Work out the finished part from the listing and answer in its coordinate system (mm). A direction names the side the tool comes from. Coordinates: 2 decimals unless noted, no trailing zeros. Order: outer loops, then holes, each group sorted by start corner. A loop starts at its lowest first (then second) coordinate and runs counter-clockwise, first axis right, second up. Notation, with made-up numbers: M 17.5,15 L 63.5,15 A19 ccw 63.5,23 Z; hole C -23.75,50.5 d11. An arc over 180 degrees is marked long. Write item = value, one per line. Start each with the question number.
Q1. Find section D-D on z = 42. Give the vertices of the cut face in (x, y), and give its area (3 significant figures).
Q2. Determine the mould class of faces 4 (the flat face through (21, 67, 30)), 5 (the flat face through (112, 35, 40)), 6 (the cylindrical face through (49.993, 60.66, 44.79)) for opening direction X: released by +X, released by -X, zero draft, split by the parting line, or undercut.
Q3. Straight lines are drawn through the part: line 1 along Y through (x, z) = (110, 7.25); line 2 along Y through (x, z) = (80, 66.75); line 3 along Y through (x, z) = (110, 24.5). For each, find the intervals that lie inside material, in ascending order.
Q4. Find section B-B on x = 30. Give the vertices of the cut face in (y, z), and give its area (3 significant figures).
Q5. Each of these flat-tipped pins is pushed along its axis until it touches: P1, Ø22, axis at x = 114.5, y = 28.5, coming from the -Z side; P2, Ø10, axis at x = 116, z = 15.5, coming from the +Y side; P3, Ø3, axis at x = 87, z = 70.5, coming from the -Y side; P4, Ø18, axis at x = 30, y = 60, coming from the +Z side. Where does it stop, or does it pass through?
Q6. Find section C-C on y = 93. Give the vertices of the cut face in (x, z), and give its area (3 significant figures).
Q7. A tool of negligible diameter and unlimited length cuts with its end or side. For faces 1 (the cylindrical face through (102, 24, 50)), 2 (the flat face through (8, 30, 37)), 3 (the flat face through (112, 95, 20)), from which of +Z, -Z, +X, -X, +Y, -Y can it reach the whole face along a straight path? Write none if from no direction.
Q8. Find section A-A on z = 57.5. Give the vertices of the cut face in (x, y), and give its area (3 significant figures).
```python
from build123d import *

# Parameters (mm, degrees)
SKETCH1_W                  = 140
SKETCH1_H                  = 120
BOSS_EXTRUDE1_DEPTH        = 60
SKETCH2_W                  = 10
SKETCH2_H                  = 60
CUT_EXTRUDE1_DEPTH         = 60
CUT_EXTRUDE2_DEPTH         = 60
SKETCH4_R                  = 10
CUT_EXTRUDE3_DEPTH         = 60
SKETCH5_R                  = 10
CUT_EXTRUDE4_DEPTH         = 60
SKETCH6_R                  = 10
CUT_EXTRUDE5_DEPTH         = 60
SKETCH7_R                  = 5
CUT_EXTRUDE6_DEPTH         = 60
SKETCH8_R                  = 10
CUT_EXTRUDE7_DEPTH         = 20
SKETCH9_R                  = 5
CUT_EXTRUDE8_DEPTH         = 47
SKETCH10_R                 = 10
CUT_EXTRUDE9_DEPTH         = 20
SKETCH11_R                 = 20
BOSS_EXTRUDE2_DEPTH        = 20
F_20_0MM_DOWEL_HOLE1_D     = 20
F_20_0MM_DOWEL_HOLE1_DEPTH = 30
F_20_0MM_DOWEL_HOLE1_TIP   = 6.00860619


with BuildPart() as part:
    # Sketch1 → Boss-Extrude1 (new body)
    with BuildSketch(Plane.XY):
        with Locations((70, 60)):
            Rectangle(SKETCH1_W, SKETCH1_H)
    extrude(amount=BOSS_EXTRUDE1_DEPTH)

    # Sketch2 → Cut-Extrude1 (cut)
    with BuildSketch(Plane.XY.offset(60)):
        with BuildLine():
            Line((140, 120), (80, 120))
            ThreePointArc((80, 120), (122.426406871, 102.426406871), (140, 60))
            Line((140, 60), (140, 120))
        make_face()
        with BuildLine():
            Line((140, 0), (140, 60))
            ThreePointArc((140, 60), (122.426406871, 17.573593129), (80, 0))
            Line((80, 0), (140, 0))
        make_face()
        with Locations((5, 60)):
            Rectangle(SKETCH2_W, SKETCH2_H)
    extrude(amount=-CUT_EXTRUDE1_DEPTH, mode=Mode.SUBTRACT)

    # Sketch3 → Cut-Extrude2 (cut)
    with BuildSketch(Plane.XY.offset(30)):
        with BuildLine():
            ThreePointArc((20, 90), (50, 60), (20, 30))
            Line((20, 30), (10, 30))
            Line((10, 30), (10, 90))
            Line((10, 90), (20, 90))
        make_face()
    extrude(amount=CUT_EXTRUDE2_DEPTH, mode=Mode.SUBTRACT)

    # Sketch4 → Cut-Extrude3 (cut)
    with BuildSketch(Plane.XY.offset(30)):
        with Locations((30, 60)):
            Circle(SKETCH4_R)
    extrude(amount=-CUT_EXTRUDE3_DEPTH, mode=Mode.SUBTRACT)

    # Sketch5 → Cut-Extrude4 (cut)
    with BuildSketch(Plane.XY.offset(20)):
        with Locations((110, 90)):
            Circle(SKETCH5_R)
    extrude(amount=-CUT_EXTRUDE4_DEPTH, mode=Mode.SUBTRACT)

    # Sketch6 → Cut-Extrude5 (cut)
    with BuildSketch(Plane.XY.offset(40)):
        with Locations((110, 90)):
            Circle(SKETCH6_R)
    extrude(amount=CUT_EXTRUDE5_DEPTH, mode=Mode.SUBTRACT)

    # Sketch7 → Cut-Extrude6 (cut)
    with BuildSketch(Plane.XY.offset(40)):
        with Locations((110, 90)):
            Circle(SKETCH7_R)
    extrude(amount=-CUT_EXTRUDE6_DEPTH, mode=Mode.SUBTRACT)

    # Sketch8 → Cut-Extrude7 (cut)
    with BuildSketch(Plane.XY.offset(60)):
        with Locations((110, 30)):
            Circle(SKETCH8_R)
    extrude(amount=-CUT_EXTRUDE7_DEPTH, mode=Mode.SUBTRACT)

    # Sketch9 → Cut-Extrude8 (cut)
    with BuildSketch(Plane.XY.offset(40)):
        with Locations((110, 30)):
            Circle(SKETCH9_R)
    extrude(amount=-CUT_EXTRUDE8_DEPTH, mode=Mode.SUBTRACT)

    # Sketch10 → Cut-Extrude9 (cut)
    with BuildSketch(Plane(origin=(0, 0, 0), x_dir=(-1, 0, 0), z_dir=(0, 0, -1))):
        with Locations((-110, 30)):
            Circle(SKETCH10_R)
    extrude(amount=-CUT_EXTRUDE9_DEPTH, mode=Mode.SUBTRACT)

    # Sketch11 → Boss-Extrude2 (add)
    with BuildSketch(Plane.XY.offset(60)):
        with Locations((80, 60)):
            Circle(SKETCH11_R)
    extrude(amount=BOSS_EXTRUDE2_DEPTH)

    # Ø20.0mm Dowel Hole1
    with Locations(Plane(origin=(80, 60, 80), x_dir=(1, 0, 0), z_dir=(0, 0, 1))):
        with Locations((0, 0)):
            Hole(F_20_0MM_DOWEL_HOLE1_D / 2, depth=F_20_0MM_DOWEL_HOLE1_DEPTH)
            with Locations((0, 0, -(F_20_0MM_DOWEL_HOLE1_DEPTH + F_20_0MM_DOWEL_HOLE1_TIP / 2))):  # 118° drill point
                Cone(0, F_20_0MM_DOWEL_HOLE1_D / 2, F_20_0MM_DOWEL_HOLE1_TIP, mode=Mode.SUBTRACT)


solid = part.part
```
Findings below:
q1.outline = M 0,0 L 80,0 A60 ccw 80,120 L 0,120 L 0,90 L 20,90 A30 cw 20,30 L 0,30 Z; hole C 110,30 d20; hole C 110,90 d20
q1.area = 12,000 mm^2
q2.face_4 = zero draft
q2.face_5 = undercut
q2.face_6 = released by -X
q3.line_1 = 8.04 to 20, 40 to 80, 100 to 111.96
q3.line_2 = 40 to 50, 70 to 80
q3.line_3 = 8.04 to 25, 35 to 85, 95 to 111.96
q4.outline = M 0,0 L 50,0 L 50,30 L 31.72,30 L 31.72,60 L 0,60 Z; M 70,0 L 120,0 L 120,60 L 88.28,60 L 88.28,30 L 70,30 Z
q4.area = 4,900 mm^2
q5.P1 = 0
q5.P2 = 111.37
q5.P3 = 40.77
q5.P4 = through
q6.outline = M 0,0 L 100.46,0 L 100.46,20 L 106,20 L 106,40 L 100.46,40 L 100.46,60 L 0,60 Z; M 114,20 L 119.54,20 L 119.54,0 L 130.11,0 L 130.11,60 L 119.54,60 L 119.54,40 L 114,40 Z
q6.area = 6,880 mm^2
q7.face_1 = +Z
q7.face_2 = +Z, -X
q7.face_3 = -Z
q8.outline = M 0,0 L 80,0 A60 ccw 80,120 L 0,120 L 0,90 L 20,90 A30 cw 20,30 L 0,30 Z; hole C 80,60 d20; hole C 110,30 d20; hole C 110,90 d20
q8.area = 11,700 mm^2
